Could you check a few things on this model? Use its own coordinates, in mm. A direction names the side the tool comes from. Coordinates: 2 decimals unless noted, no trailing zeros. Order: outer loops, then holes, each group sorted by start corner. A loop starts at its lowest first (then second) coordinate and runs counter-clockwise, first axis right, second up. Notation, with made-up numbers: M 68,-21.5 L 107,-21.5 A18 cw 107,-4.5 Z; hole C 57.25,0 d1. An arc over 180 degrees is marked long. Write item = value, one per line. Start each with the question number.
from build123d import *

# Parameters (mm, degrees)
ESQUISSE1_R             = 6
BOSS_EXTRU_1_DEPTH      = 12
ESQUISSE2_R             = 3
ENL_V_MAT_EXTRU_1_DEPTH = 12
ESQUISSE3_R             = 5
ENL_V_MAT_EXTRU_2_DEPTH = 6
ENL_V_MAT_EXTRU_3_REACH = 109.182
ESQUISSE4_R             = 2.25


with BuildPart() as part:
    # Esquisse1 → Boss.-Extru.1 (new body)
    with BuildSketch(Plane.XY):
        with BuildLine():
            Line((0, 0), (70, 0))
            Line((70, 0), (70, 37))
            ThreePointArc((70, 37), (71.464466094, 40.535533906), (75, 42))
            Line((75, 42), (83, 42))
            ThreePointArc((83, 42), (86.535533906, 43.464466094), (88, 47))
            Line((88, 47), (88, 55))
            ThreePointArc((88, 55), (86.535533906, 58.535533906), (83, 60))
            Line((83, 60), (70, 60))
            Line((70, 60), (3, 60))
            ThreePointArc((3, 60), (0.878679656, 59.121320344), (0, 57))
            Line((0, 57), (0, 0))
        make_face()
        with Locations((79, 51)):
            Circle(ESQUISSE1_R, mode=Mode.SUBTRACT)
        with BuildLine():
            Line((20, 7), (50, 7))
            ThreePointArc((50, 7), (52.121320344, 7.878679656), (53, 10))
            Line((53, 10), (53, 40))
            ThreePointArc((53, 40), (52.121320344, 42.121320344), (50, 43))
            Line((50, 43), (20, 43))
            ThreePointArc((20, 43), (17.878679656, 42.121320344), (17, 40))
            Line((17, 40), (17, 10))
            ThreePointArc((17, 10), (17.878679656, 7.878679656), (20, 7))
        make_face(mode=Mode.SUBTRACT)
    extrude(amount=BOSS_EXTRU_1_DEPTH)

    # Esquisse2 → Enlèv. mat.-Extru.1 (cut)
    with BuildSketch(Plane.XY.offset(12)):
        with Locations((12.5, 25)):
            Circle(ESQUISSE2_R)
        with Locations(Location((57.5, 25, 0), (0, 0, 180))):
            Circle(ESQUISSE2_R)
    extrude(amount=-ENL_V_MAT_EXTRU_1_DEPTH, mode=Mode.SUBTRACT)

    # Esquisse3 → Enlèv. mat.-Extru.2 (cut)
    with BuildSketch(Plane.XY.offset(12)):
        with Locations((12.5, 25)):
            Circle(ESQUISSE3_R)
        with Locations((57.5, 25)):
            Circle(ESQUISSE3_R)
    extrude(amount=-ENL_V_MAT_EXTRU_2_DEPTH, mode=Mode.SUBTRACT)

    # Esquisse4 → Enlèv. mat.-Extru.3 (cut, up to next)
    with BuildSketch(Plane.XY.offset(12), mode=Mode.PRIVATE) as enl_v_mat_extru_3_sk1:
        with Locations((11.45, 48.55)):
            Circle(ESQUISSE4_R)
    enl_v_mat_extru_3_tool1 = extrude(enl_v_mat_extru_3_sk1.sketch, amount=-ENL_V_MAT_EXTRU_3_REACH, mode=Mode.PRIVATE) & part.part
    # Esquisse4 → Enlèv. mat.-Extru.3 (cut, up to next)
    with BuildSketch(Plane.XY.offset(12), mode=Mode.PRIVATE) as enl_v_mat_extru_3_sk2:
        with Locations((58.55, 48.55)):
            Circle(ESQUISSE4_R)
    enl_v_mat_extru_3_tool2 = extrude(enl_v_mat_extru_3_sk2.sketch, amount=-ENL_V_MAT_EXTRU_3_REACH, mode=Mode.PRIVATE) & part.part
    add(enl_v_mat_extru_3_tool1.solids().sort_by_distance((11.45, 48.55, 12))[0], mode=Mode.SUBTRACT)
    add(enl_v_mat_extru_3_tool2.solids().sort_by_distance((58.55, 48.55, 12))[0], mode=Mode.SUBTRACT)


solid = part.part
(1) Imagine slicing it at A-A on y = 25. List the corners of the cut face in (x, z) for me.
(2) Please list where these lines run through material, in increasing order: probe 1 along Y at (x, z) = (12.5, 3.55); probe 2 along X at (y, z) = (47, 3.25); probe 3 along X at (y, z) = (15.5, 0.75). Write a range as from..to.
(3) For faces 1 (the flat face through (60, 23, 6)), 2 (the cylindrical face through (52.1, 7.86, 5.92)), 3 (the cylindrical face through (0.9, 59.14, 5.92)), 4 (the flat face through (70, 18, 6)), which set-ups out of +Z, -Z, +X, -X, +Y, -Y let a thin tool reach every point of the face, with its end or its side?
(4) Imagine slicing it at B-B on z = 1.75. List the corners of the cut face in (x, y) for me, plus the area to 3 significant figures.
(5) Will these pins go through, and if not, where does the flat tip stop? P1, Ø4, axis at x = 77.5, z = 8, coming from the -Y side; P2, Ø7, axis at x = 11.45, y = 48.55, coming from the -Z side; P3, Ø7.5, axis at x = 12, y = 24.5, coming from the +Z side; P4, Ø6, axis at y = 13, z = 7, coming from the +X side.
(6) Thinking about a two-plate mould opening in X: for faces 5 (the flat face through (44, 60, 6)), 6 (the flat face through (88, 51, 6)), 7 (the flat face through (10, 23, 6)), which applies, released by +X, released by -X, zero draft, split by the parting line, or undercut?
(7) Imagine slicing it at D-D on y = 39. List the corners of the cut face in (x, z) for me.
(8) Imagine slicing it at C-C on x = 45.5. List the corners of the cut face in (y, z) for me.
Response:
q1.outline = M 0,0 L 9.5,0 L 9.5,6 L 7.5,6 L 7.5,12 L 0,12 Z; M 15.5,0 L 17,0 L 17,6 L 15.5,6 Z; M 53,0 L 54.5,0 L 54.5,6 L 53,6 Z; M 60.5,0 L 70,0 L 70,12 L 62.5,12 L 62.5,6 L 60.5,6 Z
q2.probe_1 = 0..22, 28..46.56, 50.54..60
q2.probe_2 = 0..9.82, 13.08..56.92, 60.18..74.53, 83.47..88
q2.probe_3 = 0..17, 53..70
q3.face_1 = +Z
q3.face_2 = +Z, -Z
q3.face_3 = +Z, -Z, -X, +Y
q3.face_4 = +Z, -Z, +X, -Y
q4.outline = M 0,0 L 70,0 L 70,37 A5 cw 75,42 L 83,42 A5 ccw 88,47 L 88,55 A5 ccw 83,60 L 3,60 A3 ccw 0,57 Z; hole C 11.45,48.55 d4.5; hole C 12.5,25 d6; hole M 17,10 A3 ccw 20,7 L 50,7 A3 ccw 53,10 L 53,40 A3 ccw 50,43 L 20,43 A3 ccw 17,40 Z; hole C 57.5,25 d6; hole C 58.55,48.55 d4.5; hole C 79,51 d12
q4.area = 3,030 mm2
q5.P1 = 42
q5.P2 = 0
q5.P3 = 6
q5.P4 = 70
q6.face_5 = zero draft
q6.face_6 = released by +X
q6.face_7 = undercut
q7.outline = M 0,0 L 17,0 L 17,12 L 0,12 Z; M 53,0 L 70.42,0 L 70.42,12 L 53,12 Z
q8.outline = M 0,0 L 7,0 L 7,12 L 0,12 Z; M 43,0 L 60,0 L 60,12 L 43,12 Z
